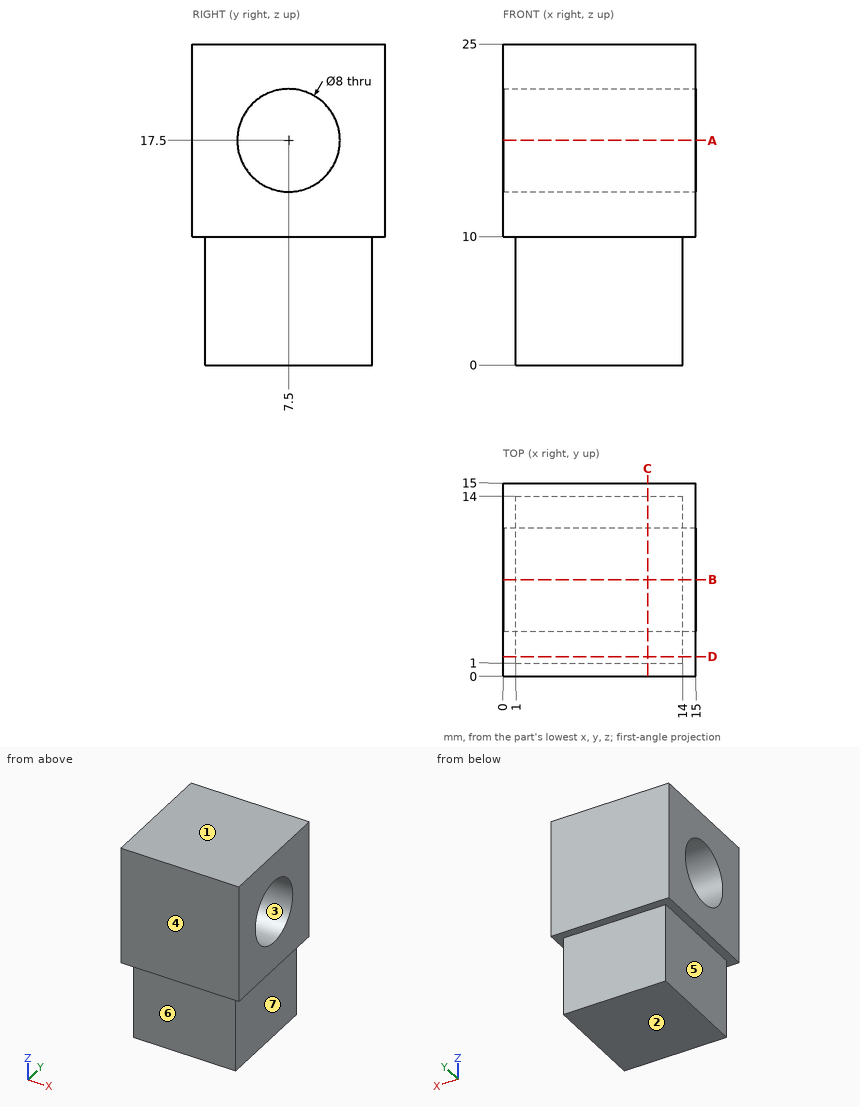
Input: dimensioned drawing with shaded views. Units: mm. Origin: part minimum x, y, z. A direction names the side the tool comes from. Give positions to 0.01 mm unless a question says otherwise; leave off trailing zeros. Loops run counter-clockwise (first coordinate to the right, second up) from the corner with the lowest first, then second, coordinate; pieces in that order, holes last. Notation, with made-up numbers: (78.5, -16.75) -> (119.5, -16.75) arc R23 cw to (119.5, 22.25) -> close; hole circle Ø11 at (57.5, 10). An arc over 180 degrees is marked (long way). Use a Markdown table: item, result.
Q1. First-contact query: P1, Ø3, axis at y = 8.5, z = 3.5, coming from the +X side; P2, Ø3, axis at x = 5, z = 5.5, coming from the -Y side. Flat tips, straight axial feed; report the tip coordinate or a pass-through.
Entries:
| item | result |
|---|---|
| P1 | stops at x = 14 |
| P2 | stops at y = 1 |
Q2. Section query B-B, the plane y = 7.5. Return the cut outline in (x, z), plus the area to 3 significant figures.
Entries:
| item | result |
|---|---|
| outline | (0, 10) -> (1, 10) -> (1, 0) -> (14, 0) -> (14, 10) -> (15, 10) -> (15, 13.5) -> (0, 13.5) -> close; (0, 21.5) -> (15, 21.5) -> (15, 25) -> (0, 25) -> close |
| area | 235 mm² |
Q3. Ray query, probe 1 along Z at (x, y) = (2.5, 7.5); probe 2 along Z at (x, y) = (2.75, 10.25); probe 3 along X at (y, z) = (2.25, 4.5). Return the intervals inside material, ascending. Write a range as from..to.
Entries:
| item | result |
|---|---|
| probe 1 | z = 0..13.5, 21.5..25 |
| probe 2 | z = 0..14.6, 20.4..25 |
| probe 3 | x = 1..14 |
Q4. Section query A-A, the plane z = 17.5. Return the cut outline in (x, y), plus the area to 3 significant figures.
Entries:
| item | result |
|---|---|
| outline | (0, 0) -> (15, 0) -> (15, 3.5) -> (0, 3.5) -> close; (0, 11.5) -> (15, 11.5) -> (15, 15) -> (0, 15) -> close |
| area | 105 mm² |
Q5. Pull-direction query (Z, two-part tool) for the marked faces 1, 2, 3 and 4; classes: pulls with the +Z half, pulls with the -Z half, needs draft (parallel to the pull), parting line crosses it, or undercut.
Entries:
| item | result |
|---|---|
| face 1 | pulls with the +Z half |
| face 2 | pulls with the -Z half |
| face 3 | undercut |
| face 4 | needs draft |
Q6. Section query C-C, the plane x = 11.25. Return the cut outline in (y, z).
Entries:
| item | result |
|---|---|
| outline | (0, 10) -> (1, 10) -> (1, 0) -> (14, 0) -> (14, 10) -> (15, 10) -> (15, 25) -> (0, 25) -> close; hole circle Ø8 at (7.5, 17.5) |
Q7. Access query for the marked faces 5, 6 and 7. Directions: +Z, -Z, +X, -X, +Y, -Y. A direction counts if a zero-diameter tool reaches every point of the face in a straight line with its end or side. Return the directions, or none.
Entries:
| item | result |
|---|---|
| face 5 | -Z, -X, +Y, -Y |
| face 6 | -Z, +X, -X, -Y |
| face 7 | -Z, +X, +Y, -Y |
Q8. Section query D-D, the plane y = 1.5. Return the cut outline in (x, z), plus the area to 3 significant figures.
Entries:
| item | result |
|---|---|
| outline | (0, 10) -> (1, 10) -> (1, 0) -> (14, 0) -> (14, 10) -> (15, 10) -> (15, 25) -> (0, 25) -> close |
| area | 355 mm² |
